```python
from build123d import *

# Parameters (mm, degrees)
CROQUIS1_W              = 24
CROQUIS1_H              = 10
CROQUIS1_R              = 1.55
SALIENTE_EXTRUIR1_DEPTH = 3
CROQUIS2_W              = 3
CROQUIS2_H              = 10
SALIENTE_EXTRUIR2_DEPTH = 15
CROQUIS3_R              = 1.55
CORTAR_EXTRUIR1_DEPTH   = 3
CROQUIS4_R              = 2.8
CORTAR_EXTRUIR2_DEPTH   = 1
CORTAR_EXTRUIR3_DEPTH   = 1
REDONDEO1_R             = 3
REDONDEO2_R             = 4


with BuildPart() as part:
    # Croquis1 → Saliente-Extruir1 (new body)
    with BuildSketch(Plane(origin=(0, 0, 0), x_dir=(1, 0, 0), z_dir=(0, 1, 0))):
        with Locations((12, 5)):
            Rectangle(CROQUIS1_W, CROQUIS1_H)
        with Locations(Location((17.5, 5, 0), (0, 0, 270))):
            Circle(CROQUIS1_R, mode=Mode.SUBTRACT)
    extrude(amount=SALIENTE_EXTRUIR1_DEPTH)

    # Croquis2 → Saliente-Extruir2 (add)
    with BuildSketch(Plane(origin=(0, 3, 0), x_dir=(1, 0, 0), z_dir=(0, 1, 0))):
        with Locations((1.5, 5)):
            Rectangle(CROQUIS2_W, CROQUIS2_H)
    extrude(amount=SALIENTE_EXTRUIR2_DEPTH)

    # Croquis3 → Cortar-Extruir1 (cut)
    with BuildSketch(Plane.ZY):
        with Locations((-5, 12.5)):
            Circle(CROQUIS3_R)
    extrude(amount=-CORTAR_EXTRUIR1_DEPTH, mode=Mode.SUBTRACT)

    # Croquis4 → Cortar-Extruir2 (cut)
    with BuildSketch(Plane(origin=(0, 3, 0), x_dir=(1, 0, 0), z_dir=(0, 1, 0))):
        with Locations(Location((17.5, 5, 0), (0, 0, 270))):
            Circle(CROQUIS4_R)
    extrude(amount=-CORTAR_EXTRUIR2_DEPTH, mode=Mode.SUBTRACT)

    # Croquis5 → Cortar-Extruir3 (cut)
    with BuildSketch(Plane(origin=(3, 0, 0), x_dir=(0, 0, -1), z_dir=(1, 0, 0))):
        Polygon((7.9, 14.174315781), (5, 15.848631561), (2.1, 14.174315781), (2.1, 10.825684219), (5, 9.151368439), (7.9, 10.825684219), align=None)
    extrude(amount=-CORTAR_EXTRUIR3_DEPTH, mode=Mode.SUBTRACT)

    # Redondeo1
    redondeo1_edges = [part.edges().sort_by_distance(p)[0] for p in [
        (1.5, 18, 0),
        (1.5, 18, -10),
        (24, 1.5, -10),
        (24, 1.5, 0),
    ]]
    fillet(redondeo1_edges, radius=REDONDEO1_R)

    # Redondeo2
    redondeo2_edges = [part.edges().sort_by_distance(p)[0] for p in [
        (3, 3, -5),
    ]]
    fillet(redondeo2_edges, radius=REDONDEO2_R)


solid = part.part
```
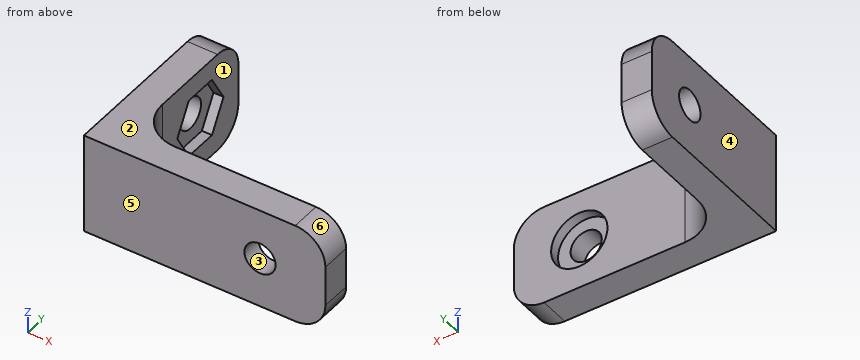
For this review, take the finished solid that the model builds, in its own axes (mm). Face numbers are marked on the shaded views. A direction names the side the tool comes from. Give positions to 0.01 mm unless a question says otherwise; leave off trailing zeros. Write each loop counter-clockwise with the first axis right and the second up, starting at its lowest first coordinate (ties: lowest second). Pieces come first, ordered by that corner, then holes. Notation, with made-up numbers: M 70,16 L 95,16 A22 cw 95,25 Z; hole C 83.5,23 d3. An arc over 180 degrees is marked long. Answer as CSV lines item,"result".
1. Draft analysis for pull direction X (two halves, no side actions). For the marked faces 3, 4, 5 and 6, state which applies: +X half, -X half, draft (parallel to the pull), parting line (faces both ways), or undercut.
Findings:
face 3,"undercut"
face 4,"-X half"
face 5,"draft"
face 6,"+X half"
2. For pin 1 (4 mm diameter, centred on x = 18.5, z = -7, fed in from -Y); pin 2 (3 mm diameter, centred on y = 7, z = -8, fed in from +X); pin 3 (3 mm diameter, centred on x = 17, z = -3.5, fed in from +Y); pin 4 (3 mm diameter, centred on y = 12.5, z = -4.5, fed in from +X), all flat-tipped, find the tip position at first contact; note any pin that passes through.
Findings:
pin 1,"stops at y = 0"
pin 2,"stops at x = 3.29"
pin 3,"stops at y = 3"
pin 4,"stops at x = 2"
3. Consider section D-D, the plane y = 15.5. Write out the cut boundary in (x, z), then the cut area to 3 significant figures.
Findings:
outline,"M 0,-9.96 L 3,-9.96 L 3,-5.6 L 2,-5.6 L 2,-4.4 L 3,-4.4 L 3,-0.04 L 0,-0.04 Z"
area,"28.5 mm2"
4. Consider section B-B, the plane x = 17.5. Write out the cut boundary in (y, z).
Findings:
outline,"M 0,-10 L 3,-10 L 3,-7.8 L 2,-7.8 L 2,-6.55 L 0,-6.55 Z; M 0,-3.45 L 2,-3.45 L 2,-2.2 L 3,-2.2 L 3,0 L 0,0 Z"
5. Wall thickness on line 1 (Z direction, x = 17.5, y = 0.4); line 2 (X direction, y = 1.2, z = -5); line 3 (X direction, y = 15.5, z = -8.25): over which ranges is each line inside the solid? List them lowest first.
Findings:
line 1,"z = -10 to -6.55, -3.45 to 0"
line 2,"x = 0 to 15.95, 19.05 to 24"
line 3,"x = 0 to 3"
6. Consider section C-C, the plane z = -1.25. Write out the cut boundary in (x, y).
Findings:
outline,"M 0,0 L 23.44,0 L 23.44,3 L 7,3 A4 cw 3,7 L 3,17.44 L 0,17.44 Z"
7. Consider section A-A, the plane y = 12.5. Write out the cut boundary in (x, z).
Findings:
outline,"M 0,-10 L 3,-10 L 3,-7.9 L 2,-7.9 L 2,-6.55 L 0,-6.55 Z; M 0,-3.45 L 2,-3.45 L 2,-2.1 L 3,-2.1 L 3,0 L 0,0 Z"
8. For the marked faces 1 and 2, list the 3-axis set-ups (+Z, -Z, +X, -X, +Y, -Y) from which the entire face can be reached by the end or side of a thin tool; tool diameter is ignored.
Findings:
face 1,"+Z, -Z, +X, +Y"
face 2,"+Z, +X, -X, +Y, -Y"
